Model file for the job. Use its own axes, mm. A direction names the side the tool comes from. Coordinates: 2 decimals unless noted, no trailing zeros. Write each loop counter-clockwise with the first axis right and the second up, starting at its lowest first coordinate (ties: lowest second). Pieces come first, ordered by that corner, then holes. Notation, with made-up numbers: (84.5, 46) - (106.5, 46) arc R28 cw to (106.5, 83) - close; hole circle Ø10 at (58.5, 7.5). An arc over 180 degrees is marked (long way). Put each result on its own line as item: value. Start each with the question number.
1. Saw through at D-D, the plane z = 1.45. Give the number of separate pieces and of enclosed holes in the cut face, plus the area to 3 significant figures.
2. Saw through at C-C, the plane y = -5. Write the cut outline in (x, z) (3 decimals).
3. Drill centre lines: L1, parallel to Y at x = 5, z = 2.7 (3 decimals); L2, parallel to Y at x = 26, z = 2.6 (3 decimals); L3, parallel to X at y = -35, z = 0.35 (3 decimals). Where is each one in solid material? Low to high. Write a range as from..to.
4. Saw through at B-B, the plane y = 8. Write the cut outline in (x, z) (3 decimals), plus the area to 4 significant figures.
5. Which spindle directions (+Z, -Z, +X, -X, +Y, -Y) get a long thin tool onto all of the face, cutting with end or side? Do faces 1 (the face through (9.785, 17, 1)), 2 (the face through (21.575, -28, 1)), 3 (the face through (-10.539, -49.257, 1.479)). Say none if no direction does.
6. Pull direction X, two halves, no side cores. Call faces 4 (the face through (28, -2.525, 1)), 5 (the face through (-11.965, -9, 1)), 6 (the face through (47.531, -49.335, 1.479)), 7 (the face through (18, -9, 0)): released by +X, released by -X, zero draft, split by the parting line, or undercut.
7. Saw through at A-A, the plane x = 24. Write the cut outline in (y, z) (3 decimals).
```python
from build123d import *

# Parameters (mm, degrees)
SKETCH001_R  = 1.7
PAD_DEPTH    = 3
POCKET_DEPTH = 10


with BuildPart() as part:
    # Sketch001 → Pad (new body)
    with BuildSketch(Plane.XY):
        with BuildLine():
            Line((-11.965, 26.939), (-11.965, -45.761))
            ThreePointArc((-11.965, -45.761), (-10.500534, -49.296534), (-6.965, -50.761))
            Line((-6.965, -50.761), (44.035, -50.761))
            ThreePointArc((44.035, -50.761), (47.570534, -49.296534), (49.035, -45.761))
            Line((49.035, -45.761), (49.035, 26.939))
            ThreePointArc((49.035, 26.939), (47.570534, 30.474534), (44.035, 31.939))
            Line((44.035, 31.939), (28.285, 31.939))
            Line((28.285, 0.939), (28.285, 31.939))
            Line((9.785, 0.939), (28.285, 0.939))
            Line((9.785, 31.939), (9.785, 0.939))
            Line((9.785, 31.939), (-6.965, 31.939))
            ThreePointArc((-6.965, 31.939), (-10.500534, 30.474534), (-11.965, 26.939))
        make_face()
        with Locations((-6.965, -45.761)):
            Circle(SKETCH001_R, mode=Mode.SUBTRACT)
        with Locations((44.035, -45.761)):
            Circle(SKETCH001_R, mode=Mode.SUBTRACT)
        with Locations((44.035, 26.939)):
            Circle(SKETCH001_R, mode=Mode.SUBTRACT)
        with Locations((-6.965, 26.939)):
            Circle(SKETCH001_R, mode=Mode.SUBTRACT)
    extrude(amount=PAD_DEPTH)

    # Sketch → Pocket (cut)
    with BuildSketch(Plane.XY):
        with BuildLine():
            Line((3.025, -2.525), (16.025, -2.525))
            ThreePointArc((16.525, -3.025), (16.378553, -2.671447), (16.025, -2.525))
            Line((16.525, -3.025), (16.525, -16.025))
            ThreePointArc((16.025, -16.525), (16.378553, -16.378553), (16.525, -16.025))
            Line((3.025, -16.525), (16.025, -16.525))
            ThreePointArc((2.525, -16.025), (2.671447, -16.378553), (3.025, -16.525))
            Line((2.525, -3.025), (2.525, -16.025))
            ThreePointArc((3.025, -2.525), (2.671447, -2.671447), (2.525, -3.025))
        make_face()
        with BuildLine():
            Line((22.075, -2.525), (35.075, -2.525))
            ThreePointArc((35.575, -3.025), (35.428553, -2.671447), (35.075, -2.525))
            Line((35.575, -3.025), (35.575, -16.025))
            ThreePointArc((35.075, -16.525), (35.428553, -16.378553), (35.575, -16.025))
            Line((22.075, -16.525), (35.075, -16.525))
            ThreePointArc((21.575, -16.025), (21.721447, -16.378553), (22.075, -16.525))
            Line((21.575, -3.025), (21.575, -16.025))
            ThreePointArc((22.075, -2.525), (21.721447, -2.671447), (21.575, -3.025))
        make_face()
        with BuildLine():
            Line((3.025, -21.575), (16.025, -21.575))
            ThreePointArc((16.525, -22.075), (16.378553, -21.721447), (16.025, -21.575))
            Line((16.525, -22.075), (16.525, -35.075))
            ThreePointArc((16.025, -35.575), (16.378553, -35.428553), (16.525, -35.075))
            Line((3.025, -35.575), (16.025, -35.575))
            ThreePointArc((2.525, -35.075), (2.671447, -35.428553), (3.025, -35.575))
            Line((2.525, -22.075), (2.525, -35.075))
            ThreePointArc((3.025, -21.575), (2.671447, -21.721447), (2.525, -22.075))
        make_face()
        with BuildLine():
            Line((22.075, -21.575), (35.075, -21.575))
            ThreePointArc((35.575, -22.075), (35.428553, -21.721447), (35.075, -21.575))
            Line((35.575, -22.075), (35.575, -35.075))
            ThreePointArc((35.075, -35.575), (35.428553, -35.428553), (35.575, -35.075))
            Line((22.075, -35.575), (35.075, -35.575))
            ThreePointArc((21.575, -35.075), (21.721447, -35.428553), (22.075, -35.575))
            Line((21.575, -22.075), (21.575, -35.075))
            ThreePointArc((22.075, -21.575), (21.721447, -21.721447), (21.575, -22.075))
        make_face()
    extrude(amount=POCKET_DEPTH, mode=Mode.SUBTRACT)


solid = part.part
```
Final values:
1. separate pieces: 1
1. enclosed holes: 8
1. area: 3,630 mm²
2. outline: (-11.965, 0) - (2.525, 0) - (2.525, 3) - (-11.965, 3) - close; (16.525, 0) - (21.575, 0) - (21.575, 3) - (16.525, 3) - close; (35.575, 0) - (49.035, 0) - (49.035, 3) - (35.575, 3) - close
3. L1: y = -50.761..-35.575, -21.575..-16.525, -2.525..31.939
3. L2: y = -50.761..-35.575, -21.575..-16.525, -2.525..0.939
3. L3: x = -11.965..2.525, 16.525..21.575, 35.575..49.035
4. outline: (-11.965, 0) - (9.785, 0) - (9.785, 3) - (-11.965, 3) - close; (28.285, 0) - (49.035, 0) - (49.035, 3) - (28.285, 3) - close
4. area: 127.5 mm²
5. face 1: +Z, -Z, +Y
5. face 2: +Z, -Z
5. face 3: +Z, -Z, -X, -Y
6. face 4: undercut
6. face 5: released by -X
6. face 6: released by +X
6. face 7: zero draft
7. outline: (-50.761, 0) - (-35.575, 0) - (-35.575, 3) - (-50.761, 3) - close; (-21.575, 0) - (-16.525, 0) - (-16.525, 3) - (-21.575, 3) - close; (-2.525, 0) - (0.939, 0) - (0.939, 3) - (-2.525, 3) - close
